Input: part model. Units: mm. Frame: model coordinates. A direction names the side the tool comes from. Round coordinates to 2 decimals unless told otherwise and drop trailing zeros. Order: outer loops, then holes, each group sorted by start corner. A loop starts at its lowest first (then second) coordinate and runs counter-clockwise, first axis right, second up.
Item 1: Reachability of faces 4 (the flat face through (-30, 23, 21)), 5 (the flat face through (38, 11, 21)), 6 (the flat face through (22, -10, 21)) from +Z, -Z, +X, -X, +Y, -Y: full face, straight path, thin tool, end or side. Return the list, or none.
Item 2: Mould query, pull axis Z, two halves, no side actions, for faces 1 (the cylindrical face through (-41.7, 0.2, 10.9)), 2 (the flat face through (-22, 44, 21)), 3 (the flat face through (1, 7, 0)). Classes: released by +Z, released by -Z, zero draft, split by the parting line, or undercut.
Item 3: Cut plane B-B on x = -38.5. Output: boundary loops of the cut face in (y, z), then the cut area to 3 significant figures.
Item 4: Cut plane D-D on z = 13.5. Output: boundary loops of the cut face in (x, y).
Item 5: First-contact query: pin 1 (4 mm diameter, centred on x = 19, z = 17.5, fed in from +Y); pin 2 (18.5 mm diameter, centred on x = 38, z = 13.5, fed in from +Y); pin 3 (1 mm diameter, centred on x = 29.5, y = 7.5, fed in from -Z); pin 4 (18.5 mm diameter, centred on x = -39, z = 22, fed in from +Y). Flat tips, straight axial feed; report the tip coordinate or a pass-through.
Item 6: Cut plane A-A on z = 8.5. Output: boundary loops of the cut face in (x, y), then the cut area to 3 significant figures.
Item 7: Line query: L1, parallel to Z at x = 38.5, y = -4.75; L2, parallel to X at y = -4.5, z = 8.5; L3, parallel to X at y = 24, z = 37.5. Output: solid intervals per line, ascending.
Item 8: Cut plane C-C on y = 23.5. Output: boundary loops of the cut face in (x, z).
```python
from build123d import *

# Parameters (mm, degrees)
DODANIE_WYCI_GNI_CIE1_DEPTH = 42
SZKIC2_R                    = 9.5
WYTNIJ_WYCI_GNI_CIE1_DEPTH  = 42
SZKIC3_R                    = 4
WYTNIJ_WYCI_GNI_CIE2_DEPTH  = 22


with BuildPart() as part:
    # Szkic1 → Dodanie-wyciągnięcie1 (new body)
    with BuildSketch(Plane.XY):
        Polygon((-47, 11), (-30, 11), (-30, 36), (-13, 53), (13, 53), (30, 36), (30, 11), (47, 11), (47, -11), (23, -11), (21, -9), (-21, -9), (-23, -11), (-47, -11), align=None)
    extrude(amount=DODANIE_WYCI_GNI_CIE1_DEPTH)

    # Szkic2 → Wytnij-wyciągnięcie1 (cut)
    with BuildSketch(Plane(origin=(0, 0, 0), x_dir=(-1, 0, 0), z_dir=(0, 0, -1))):
        with Locations((0, 23.5)):
            Circle(SZKIC2_R)
    extrude(amount=-WYTNIJ_WYCI_GNI_CIE1_DEPTH, mode=Mode.SUBTRACT)

    # Szkic3 → Wytnij-wyciągnięcie2 (cut)
    with BuildSketch(Plane(origin=(0, 11, 0), x_dir=(1, 0, 0), z_dir=(0, 1, 0))):
        with Locations((-38.5, -8.5)):
            Circle(SZKIC3_R)
        with Locations((-38.5, -33.5)):
            Circle(SZKIC3_R)
        with Locations((38.5, -33.5)):
            Circle(SZKIC3_R)
        with Locations((38.5, -8.5)):
            Circle(SZKIC3_R)
    extrude(amount=-WYTNIJ_WYCI_GNI_CIE2_DEPTH, mode=Mode.SUBTRACT)


solid = part.part
```
From the geometry:
1. face 4: +Z, -Z, -X, +Y
1. face 5: +Z, -Z, +X, +Y
1. face 6: +Z, -Z, -Y
2. face 1: undercut
2. face 2: zero draft
2. face 3: released by -Z
3. outline: (-11, 0) - (11, 0) - (11, 4.5) - (-11, 4.5) - close; (-11, 12.5) - (11, 12.5) - (11, 29.5) - (-11, 29.5) - close; (-11, 37.5) - (11, 37.5) - (11, 42) - (-11, 42) - close
3. area: 572 mm2
4. outline: (-47, -11) - (-23, -11) - (-21, -9) - (21, -9) - (23, -11) - (47, -11) - (47, 11) - (30, 11) - (30, 36) - (13, 53) - (-13, 53) - (-30, 36) - (-30, 11) - (-47, 11) - close; hole circle Ø19 at (0, 23.5)
5. pin 1: stops at y = 49
5. pin 2: stops at y = 37.25
5. pin 3: stops at z = 0
5. pin 4: stops at y = 36.25
6. outline: (-47, -11) - (-42.5, -11) - (-42.5, 11) - (-47, 11) - close; (-34.5, -11) - (-23, -11) - (-21, -9) - (21, -9) - (23, -11) - (34.5, -11) - (34.5, 11) - (30, 11) - (30, 36) - (13, 53) - (-13, 53) - (-30, 36) - (-30, 11) - (-34.5, 11) - close; (42.5, -11) - (47, -11) - (47, 11) - (42.5, 11) - close; hole circle Ø19 at (0, 23.5)
6. area: 3,580 mm2
7. L1: z = 0 to 4.5, 12.5 to 29.5, 37.5 to 42
7. L2: x = -47 to -42.5, -34.5 to 34.5, 42.5 to 47
7. L3: x = -30 to -9.49, 9.49 to 30
8. outline: (-30, 0) - (-9.5, 0) - (-9.5, 42) - (-30, 42) - close; (9.5, 0) - (30, 0) - (30, 42) - (9.5, 42) - close
